```python
from build123d import *

# Parameters (mm, degrees)
CROQUIS1_W              = 127.5
CROQUIS1_H              = 40
SALIENTE_EXTRUIR2_DEPTH = 135
CROQUIS3_W              = 119.7
CROQUIS3_H              = 29.7
SALIENTE_EXTRUIR3_DEPTH = 10
CORTAR_EXTRUIR1_DEPTH   = 184
CORTAR_EXTRUIR2_DEPTH   = 184
VACIADO1_T              = -5


with BuildPart() as part:
    # Croquis1 → Saliente-Extruir2 (new body)
    with BuildSketch(Plane.XY):
        Rectangle(CROQUIS1_W, CROQUIS1_H)
    extrude(amount=SALIENTE_EXTRUIR2_DEPTH)

    # Croquis3 → Saliente-Extruir3 (add)
    with BuildSketch(Plane(origin=(0, 0, 0), x_dir=(-1, 0, 0), z_dir=(0, 0, -1))):
        with Locations((-1.25, 0)):
            Rectangle(CROQUIS3_W, CROQUIS3_H)
    extrude(amount=SALIENTE_EXTRUIR3_DEPTH)

    # Croquis4 → Cortar-Extruir1 (cut)
    with BuildSketch(Plane.ZY.offset(63.75)):
        Polygon((135, 20), (20, 20), (135, -13), align=None)
    extrude(amount=-CORTAR_EXTRUIR1_DEPTH, mode=Mode.SUBTRACT)

    # Croquis5 → Cortar-Extruir2 (cut)
    with BuildSketch(Plane(origin=(0, 20, 0), x_dir=(1, 0, 0), z_dir=(0, 1, 0))):
        Polygon((-63.75, -20), (-15, -135), (15, -135), (63.75, -20), (107.189901301, -122.473613325), (58.694004086, -179.25211437), (-87.283869917, -146.849702978), align=None)
    extrude(amount=-CORTAR_EXTRUIR2_DEPTH, mode=Mode.SUBTRACT)

    # Vaciado1
    vaciado1_openings = [part.faces().sort_by_distance(p)[0] for p in [
        (0, -20, 53.411416263),
    ]]
    offset(amount=VACIADO1_T, openings=vaciado1_openings, kind=Kind.INTERSECTION)


solid = part.part
```
Design review of the part built by this model. Coordinates are the model's own, in mm. A direction names the side the tool comes from. Coordinates: 2 decimals unless noted, no trailing zeros. Loops run counter-clockwise (first coordinate to the right, second up) from the corner with the lowest first, then second, coordinate; pieces in that order, holes last. Notation, with made-up numbers: (-19, 67.25) -> (21, 67.25) arc R23 cw to (21, 87.25) -> close; hole circle Ø8 at (62.25, 47). An arc over 180 degrees is marked (long way). Answer as a JSON object with one key per item and string values.
Q1. To check wall thickness, follow L1, parallel to X at y = 3, z = 5.5; L2, parallel to X at y = 2.5, z = 1.5; L3, parallel to Y at x = -56, z = 7. State the ranges of each line that lie inside material, in increasing order.
Answer block:
{"L1": "x = -63.75 to -58.75, 58.75 to 63.75", "L2": "x = -63.75 to -53.6, 56.1 to 63.75", "L3": "y = 15 to 20"}
Q2. The part is to be moulded in two halves that separate along Y. For faces 6 (the flat face through (-1, 20, 10)), 7 (the flat face through (2, -9.85, 0)), 8 (the flat face through (2, 0, -5)), 9 (the flat face through (2, 0, -10)), say which applies: +Y half, -Y half, draft (parallel to the pull), parting line (faces both ways), or undercut.
Answer block:
{"face 6": "+Y half", "face 7": "undercut", "face 8": "undercut", "face 9": "draft"}
Q3. Take a section at A-A on y = -2. Give the boundary of the cut face in (x, z), plus the area to 3 significant figures.
Answer block:
{"outline": "(-63.75, 0) -> (-58.6, 0) -> (-58.6, -10) -> (61.1, -10) -> (61.1, 0) -> (63.75, 0) -> (63.75, 20) -> (31.25, 96.67) -> (-31.25, 96.67) -> (-63.75, 20) -> close; hole (-58.75, 5) -> (-53.6, 5) -> (-53.6, -5) -> (56.1, -5) -> (56.1, 5) -> (58.75, 5) -> (58.75, 18.98) -> (33.5, 78.54) -> (-33.5, 78.54) -> (-58.75, 18.98) -> close", "area": "2,800 mm^2"}
Q4. Tool access review of faces 1 (the flat face through (-53.6, 0, 0)), 2 (the flat face through (61.1, 0, -5)), 3 (the flat face through (-0.892, 7.398, 63.917)), 4 (the flat face through (2, -14.85, -5)), 5 (the flat face through (58.75, -3, 12)): name each direction out of +Z, -Z, +X, -X, +Y, -Y from which nothing blocks a thin tool from reaching the whole face with its end or side.
Answer block:
{"face 1": "none", "face 2": "-Z, +X, +Y, -Y", "face 3": "+Z, +X, -X, +Y", "face 4": "-Z, +X, -X, -Y", "face 5": "-Y"}
Q5. Take a section at B-B on z = 29.5. Give the boundary of the cut face in (x, y), plus the area to 3 significant figures.
Answer block:
{"outline": "(-59.72, -20) -> (-54.29, -20) -> (-54.29, 12.07) -> (54.29, 12.07) -> (54.29, -20) -> (59.72, -20) -> (59.72, 17.27) -> (-59.72, 17.27) -> close", "area": "970 mm^2"}
Q6. Take a section at D-D on y = 13. Give the boundary of the cut face in (x, z), plus the area to 3 significant figures.
Answer block:
{"outline": "(-63.75, 0) -> (-58.6, 0) -> (-58.6, -10) -> (61.1, -10) -> (61.1, 0) -> (63.75, 0) -> (63.75, 20) -> (53.41, 44.39) -> (-53.41, 44.39) -> (-63.75, 20) -> close; hole (-58.75, 5) -> (58.75, 5) -> (58.75, 18.98) -> (55.66, 26.27) -> (-55.66, 26.27) -> (-58.75, 18.98) -> close", "area": "4,130 mm^2"}
Q7. Clearance check with flat-ended pins moving along their axes: pin 1 Ø3 at (x, z) = (-18.5, -6.5) entering from +Y; pin 2 Ø3 at (x, y) = (49.5, -14.5) entering from +Z; pin 3 Ø1 at (y, z) = (-4, 49) entering from +X. State where each tip first meets the part, or that it passes through.
Answer block:
{"pin 1": "stops at y = 14.85", "pin 2": "stops at z = 57.15", "pin 3": "stops at x = 51.67"}
Q8. Take a section at C-C on x = 1.5. Give the boundary of the cut face in (y, z).
Answer block:
{"outline": "(-20, 0) -> (-14.85, 0) -> (-14.85, -10) -> (14.85, -10) -> (14.85, 0) -> (20, 0) -> (20, 20) -> (-13, 135) -> (-20, 135) -> (-20, 130) -> (-16.77, 130) -> (15, 19.3) -> (15, 5) -> (9.85, 5) -> (9.85, -5) -> (-9.85, -5) -> (-9.85, 5) -> (-20, 5) -> close"}
